Work out the finished part from the listing and answer in its coordinate system (mm). A direction names the side the tool comes from. Coordinates: 2 decimals unless noted, no trailing zeros. Order: outer loops, then holes, each group sorted by start corner. A loop starts at its lowest first (then second) coordinate and runs counter-clockwise, first axis right, second up.
1. Determine the mould class of faces 5 (the cylindrical face through (-1320.416, 626.178, 23.811)), 6 (the flat face through (-1144.463, 677.245, 12.567)), 7 (the flat face through (-941.145, 698, 13)) for opening direction Y: +Y half, -Y half, draft (parallel to the pull), parting line (faces both ways), or undercut.
2. The part is cut by section C-C, the plane x = -1097.5. Give the vertices of the cut face in (y, z) (3 decimals).
3. The part is cut by section B-B, the plane y = 669. Give the vertices of the cut face in (x, z) (3 decimals), then the cut area to 3 significant figures.
4. Find the intervals of material crossed by probe 1 along Z at (x, y) = (-1155.5, 701) (3 decimals); probe 2 along Y at (x, z) = (-1287.5, 18); probe 3 along X at (y, z) = (607, 23.75), in increasing order.
5. The part is cut by section D-D, the plane y = 750.5. Give the vertices of the cut face in (x, z) (3 decimals).
6. The part is cut by section A-A, the plane z = 18.25. Give the vertices of the cut face in (x, y), then the cut area to 3 significant figures.
7. Flat-ended cylindrical pins translate along their axes: pin 1 Ø12 at (x, y) = (-1265, 622) entering from -Z; pin 2 Ø2 at (y, z) = (644, 16) entering from -X; pin 3 Ø10 at (y, z) = (763, 10) entering from -X; pin 4 Ø5.5 at (y, z) = (719.5, 13) entering from -X. Find the tip coordinate at first contact, or state that the pin passes through.
8. A tool of negligible diameter and unlimited length cuts with its end or side. For faces 1 (the flat face through (-1134, 594.743, 13)), 2 (the flat face through (-967, 713, 3.175)), 3 (the flat face through (-1168, 711, 22.225)), 4 (the flat face through (-1049.535, 680.905, 12.522)), from which of +Z, -Z, +X, -X, +Y, -Y can it reach the whole face along a straight path? Write none if from no direction.
```python
from build123d import *

# Parameters (mm, degrees)
SKETCH1_R           = 14.2875
SKETCH1_R_2         = 25.4
BOSS_EXTRUDE3_DEPTH = 25.4
SKETCH9_R           = 14.2875
CUT_EXTRUDE7_DEPTH  = 1537.409158581
SKETCH10_W          = 19.05
SKETCH10_H          = 44.45
CUT_EXTRUDE8_DEPTH  = 871.429558372
SKETCH11_W          = 44.45
SKETCH11_H          = 19.05
CUT_EXTRUDE9_DEPTH  = 139.835175171
SKETCH13_R          = 14.2875
BOSS_EXTRUDE4_DEPTH = 25.4
SKETCH14_W          = 44.45
SKETCH14_H          = 19.05
CUT_EXTRUDE10_DEPTH = 81.475845846
FILLET3_R           = 25.4


with BuildPart() as part:
    # Sketch1 → Boss-Extrude3 (new body)
    # profile 1 of 13: a face of its own
    with BuildSketch(Plane.XY):
        with BuildLine():
            ThreePointArc((-1322.144654144, 616.967775532), (-1314.705166386, 634.928287774), (-1296.744654144, 642.367775532))
            Line((-1296.744654144, 642.367775532), (-1322.144654144, 642.367775532))
            Line((-1322.144654144, 642.367775532), (-1322.144654144, 616.967775532))
        make_face()
    # profile 2 of 13: a face of its own
    with BuildSketch(Plane.XY):
        with BuildLine():
            ThreePointArc((-1296.744654144, 591.567775532), (-1314.705166386, 599.00726329), (-1322.144654144, 616.967775532))
            Line((-1322.144654144, 616.967775532), (-1322.144654144, 591.567775532))
            Line((-1322.144654144, 591.567775532), (-1296.744654144, 591.567775532))
        make_face()
    # profile 3 of 13: a face of its own
    with BuildSketch(Plane.XY):
        with BuildLine():
            ThreePointArc((-1258.644654144, 616.967775532), (-1261.152687268, 630.562697152), (-1268.34659083, 642.367775532))
            Line((-1268.34659083, 642.367775532), (-1296.744654144, 642.367775532))
            ThreePointArc((-1296.744654144, 642.367775532), (-1278.784141902, 634.928287774), (-1271.344654144, 616.967775532))
            ThreePointArc((-1271.344654144, 616.967775532), (-1278.784141902, 599.00726329), (-1296.744654144, 591.567775532))
            Line((-1296.744654144, 591.567775532), (-1268.34659083, 591.567775532))
            ThreePointArc((-1268.34659083, 591.567775532), (-1261.152687268, 603.372853911), (-1258.644654144, 616.967775532))
        make_face()
    # profile 4 of 13: a face of its own
    with BuildSketch(Plane.XY):
        with BuildLine():
            Line((-1166.346089039, 600.519446439), (-1195.144654144, 642.367775532))
            Line((-1195.144654144, 642.367775532), (-1268.34659083, 642.367775532))
            ThreePointArc((-1268.34659083, 642.367775532), (-1261.152687268, 630.562697152), (-1258.644654144, 616.967775532))
            ThreePointArc((-1258.644654144, 616.967775532), (-1261.152687268, 603.372853911), (-1268.34659083, 591.567775532))
            Line((-1268.34659083, 591.567775532), (-1128.284013271, 591.567775532))
            Line((-1128.284013271, 591.567775532), (-1128.284013271, 626.712443646))
            Line((-1128.284013271, 626.712443646), (-1166.346089039, 600.519446439))
        make_face()
    # profile 5 of 13: a face of its own
    with BuildSketch(Plane.XY):
        Polygon((-1128.284013271, 642.367775532), (-1195.144654144, 642.367775532), (-1166.346089039, 600.519446439), (-1128.284013271, 626.712443646), align=None)
    # profile 6 of 13: a face of its own
    with BuildSketch(Plane.XY):
        Polygon((-991.944654144, 720.536450369), (-991.944654144, 782.202950703), (-1195.144654144, 642.367775532), (-1128.284013271, 642.367775532), (-1105.534633972, 642.367775532), align=None)
    # profile 7 of 13: a face of its own
    with BuildSketch(Plane.XY):
        Polygon((-1105.534633972, 642.367775532), (-1128.284013271, 642.367775532), (-1128.284013271, 626.712443646), align=None)
    # profile 8 of 13: a face of its own
    with BuildSketch(Plane.XY):
        Polygon((-941.144654144, 591.567775532), (-941.144654144, 642.367775532), (-991.944654144, 642.367775532), (-1105.534633972, 642.367775532), (-1128.284013271, 626.712443646), (-1128.284013271, 591.567775532), align=None)
        with Locations((-966.544654144, 616.967775532)):
            Circle(SKETCH1_R, mode=Mode.SUBTRACT)
    # profile 9 of 13: a face of its own
    with BuildSketch(Plane.XY):
        Polygon((-941.144654144, 782.202950703), (-991.944654144, 782.202950703), (-963.146089039, 740.354621609), (-991.944654144, 720.536450369), (-991.944654144, 642.367775532), (-941.144654144, 642.367775532), align=None)
    # profile 10 of 13: a face of its own
    with BuildSketch(Plane.XY):
        Polygon((-963.146089039, 740.354621609), (-991.944654144, 782.202950703), (-991.944654144, 720.536450369), align=None)
    # profile 11 of 13: a face of its own
    with BuildSketch(Plane.XY):
        with Locations((-966.544654144, 616.967775532)):
            Circle(SKETCH1_R)
    # profile 12 of 13: a face of its own
    with BuildSketch(Plane.XY):
        with Locations((-1296.744654144, 616.967775532)):
            Circle(SKETCH1_R_2)
        with Locations((-1296.744654144, 616.967775532)):
            Circle(SKETCH1_R, mode=Mode.SUBTRACT)
    # profile 13 of 13: a face of its own
    with BuildSketch(Plane.XY):
        with Locations((-1296.744654144, 616.967775532)):
            Circle(SKETCH1_R)
    extrude(amount=BOSS_EXTRUDE3_DEPTH)

    # Sketch9 → Cut-Extrude7 (cut, through all)
    with BuildSketch(Plane.XY.offset(25.4)):
        with Locations((-1296.744654144, 616.967775532)):
            Circle(SKETCH9_R)
        with Locations((-966.544654144, 616.967775532)):
            Circle(SKETCH9_R)
    extrude(amount=-CUT_EXTRUDE7_DEPTH, mode=Mode.SUBTRACT)

    # Sketch10 → Cut-Extrude8 (cut, through all)
    with BuildSketch(Plane.ZY.offset(1322.144654144)):
        with Locations((12.7, 616.967775532)):
            Rectangle(SKETCH10_W, SKETCH10_H)
    extrude(amount=-CUT_EXTRUDE8_DEPTH, mode=Mode.SUBTRACT)

    # Sketch11 → Cut-Extrude9 (cut)
    with BuildSketch(Plane(origin=(0, 782.202950703, 0), x_dir=(1, 0, 0), z_dir=(0, 1, 0))):
        with Locations((-966.544654144, -12.7)):
            Rectangle(SKETCH11_W, SKETCH11_H)
    extrude(amount=-CUT_EXTRUDE9_DEPTH, mode=Mode.SUBTRACT)

    # Sketch13 → Boss-Extrude4 (add)
    # profile 1 of 2: a face of its own
    with BuildSketch(Plane.XY):
        with BuildLine():
            Line((-1169.471208218, 758.939487681), (-1211.319537311, 730.140922576))
            Line((-1211.319537311, 730.140922576), (-1180.283016907, 685.040532503))
            ThreePointArc((-1180.283016907, 685.040532503), (-1154.1022052, 692.46774594), (-1139.555223473, 715.467392104))
            Line((-1139.555223473, 715.467392104), (-1169.471208218, 758.939487681))
        make_face()
        with Locations((-1176.905095286, 722.990494894)):
            Circle(SKETCH13_R, mode=Mode.SUBTRACT)
    # profile 2 of 2: a face of its own
    with BuildSketch(Plane.XY):
        with BuildLine():
            ThreePointArc((-1139.555223473, 715.467392104), (-1154.1022052, 692.46774594), (-1180.283016907, 685.040532503))
            Line((-1180.283016907, 685.040532503), (-1165.130807959, 663.022260959))
            Line((-1165.130807959, 663.022260959), (-1123.282478866, 691.820826065))
            Line((-1123.282478866, 691.820826065), (-1139.555223473, 715.467392104))
        make_face()
    extrude(amount=BOSS_EXTRUDE4_DEPTH)

    # Sketch14 → Cut-Extrude10 (cut)
    with BuildSketch(Plane(origin=(-730.269249407, 1061.183005622, 0), x_dir=(0.8237860057708082, 0.5669008878950341, 0), z_dir=(-0.5669008878950341, 0.8237860057708082, 0))):
        with Locations((-558.550546057, -12.7)):
            Rectangle(SKETCH14_W, SKETCH14_H)
    extrude(amount=-CUT_EXTRUDE10_DEPTH, mode=Mode.SUBTRACT)

    # Fillet3
    # the kernel refuses this fillet: 25.4 mm, written as the material it takes off along each edge
    with BuildSketch(Plane(origin=(-941.144654144, 591.567775532, -63.5), x_dir=(-1, 0, 0), z_dir=(0, 0, 1)), Plane(origin=(-1322.144654144, 591.567775532, -63.5), x_dir=(0, 1, 0), z_dir=(0, 0, 1)), Plane(origin=(-1322.144654144, 642.367775532, -63.5), x_dir=(1, 0, 0), z_dir=(0, 0, 1))) as fillet3_piece_1:
        with BuildLine():
            CenterArc((FILLET3_R, -FILLET3_R), FILLET3_R, 90, 90)
            Line((0, -FILLET3_R), (0, 0))
            Line((0, 0), (FILLET3_R, 0))
        make_face()
    extrude(amount=152.4, mode=Mode.SUBTRACT)


solid = part.part
```
Geometry says:
1. face 5: parting line
1. face 6: undercut
1. face 7: draft
2. outline: (591.568, 0) - (642.368, 0) - (642.368, 25.4) - (591.568, 25.4) - close; (647.897, 0) - (709.563, 0) - (709.563, 25.4) - (647.897, 25.4) - close; hole (594.743, 3.175) - (639.193, 3.175) - (639.193, 22.225) - (594.743, 22.225) - close
3. outline: (-1169.244, 0) - (-1066.834, 0) - (-1066.834, 25.4) - (-1169.244, 25.4) - close; (-991.945, 0) - (-941.145, 0) - (-941.145, 25.4) - (-991.945, 25.4) - close; hole (-1165.39, 3.175) - (-1156.444, 3.175) - (-1156.444, 22.225) - (-1165.39, 22.225) - close; hole (-988.77, 3.175) - (-944.32, 3.175) - (-944.32, 22.225) - (-988.77, 22.225) - close
3. area: 2,870 mm2
4. probe 1: z = 0 to 3.175, 22.225 to 25.4
4. probe 2: y = 591.57 to 594.74, 639.19 to 642.37
4. probe 3: x = -1320.11 to -1306.98, -1286.51 to -976.78, -956.31 to -943.18
5. outline: (-1181.735, 0) - (-1163.663, 0) - (-1163.663, 25.4) - (-1181.735, 25.4) - (-1181.735, 22.225) - (-1167.518, 22.225) - (-1167.518, 3.175) - (-1181.735, 3.175) - close; (-1038.013, 0) - (-941.145, 0) - (-941.145, 25.4) - (-1038.013, 25.4) - close; hole (-988.77, 3.175) - (-944.32, 3.175) - (-944.32, 22.225) - (-988.77, 22.225) - close
6. outline: (-1309.04, 594.74) arc R25.4 ccw to (-1296.74, 591.57) - (-966.54, 591.57) arc R25.4 ccw to (-954.25, 594.74) - close; (-1309.04, 639.19) - (-941.14, 639.19) - (-941.14, 782.2) - (-944.32, 782.2) - (-944.32, 642.37) - (-988.77, 642.37) - (-988.77, 782.2) - (-991.94, 782.2) - (-1123.28, 691.82) - (-1169.47, 758.94) - (-1172.09, 757.14) - (-1125.9, 690.02) - (-1162.52, 664.82) - (-1208.7, 731.94) - (-1211.32, 730.14) - (-1165.13, 663.02) - (-1195.14, 642.37) - (-1296.74, 642.37) arc R25.4 ccw to start; hole (-1105.53, 642.37) - (-991.94, 642.37) - (-991.94, 720.54) - close
6. area: 13,400 mm2
7. pin 1: stops at z = 0
7. pin 2: stops at x = -1194.23
7. pin 3: stops at x = -1170.84
7. pin 4: stops at x = -1205.89
8. face 1: +X, -X
8. face 2: +Y
8. face 3: none
8. face 4: +Z, -Z
